```python
from build123d import *

# Parameters (mm, degrees)
SKETCH2_R          = 2.5
SKETCH2_R_2        = 2.2
SKETCH3_W          = 7.732538493
SKETCH3_H          = 7
CUT_EXTRUDE1_DEPTH = 5


with BuildPart() as part:
    # Sweep1: sweep along a path in Sketch1
    with BuildLine(Plane(origin=(0, 0, 0), x_dir=(0, 0, -1), z_dir=(1, 0, 0))) as sweep1_path:
        Line((0, 23), (-3, 23))
        ThreePointArc((-3, 23), (-15.57477634, 19.956594203), (-25.366269246, 11.5))
        ThreePointArc((-25.366269246, 11.5), (-31.811636627, 5.077357788), (-40, 1.10951216))
        ThreePointArc((-40, 1.10951216), (-43.826672111, 0.278791213), (-47.732538493, 0))
    # Sketch2 → Sweep1 (sweep)
    with BuildSketch(Plane.XY):
        with Locations((0, 23)):
            Circle(SKETCH2_R)
        with Locations((0, 23)):
            Circle(SKETCH2_R_2, mode=Mode.SUBTRACT)
    sweep(path=sweep1_path.line)

    # Sketch3 → Cut-Extrude1 (cut, symmetric)
    with BuildSketch(Plane(origin=(0, 0, 0), x_dir=(0, 0, -1), z_dir=(1, 0, 0))):
        with Locations((-43.866269246, 1)):
            Rectangle(SKETCH3_W, SKETCH3_H)
    extrude(amount=CUT_EXTRUDE1_DEPTH, both=True, mode=Mode.SUBTRACT)

    # Sketch4 → Revolve1 (revolve)
    with BuildSketch(Plane(origin=(0, 0, 0), x_dir=(0, 0, -1), z_dir=(1, 0, 0)), mode=Mode.PRIVATE) as revolve1_sk:
        with BuildLine():
            Line((0, 25.2), (0, 25.5))
            ThreePointArc((0, 25.5), (1.13447358, 25.928498418), (1.702386917, 27))
            Line((1.702386917, 27), (2, 26.962231588))
            ThreePointArc((2, 26.962231588), (1.332803452, 25.703408965), (0, 25.2))
        make_face()
    revolve(revolve1_sk.sketch.rotate(Axis((0, 23, 0), (0, 0, -1)), 90), axis=Axis((0, 23, 0), (0, 0, -1)))


solid = part.part
```
Source: CAD feature listing. Evaluate the final solid. Frame: model axes, mm. Round coordinates to 2 decimals unless told otherwise and drop trailing zeros. Write each loop counter-clockwise with the first axis right and the second up, starting at its lowest first coordinate (ties: lowest second). Pieces come first, ordered by that corner, then holes. Notation, with made-up numbers: M -14.5,71 L 24.5,71 A21 cw 24.5,108 Z; hole C -4,-11 d5. An arc over 180 degrees is marked long. Use CSV: the item, a comma, the result in double quotes. Start each with the question number.
Q1. Cut plane B-B on y = 19.5. Count the separate pieces of the cut face and the enclosed holes in it, plus the area to 3 significant figures.
Q2. Cut plane A-A on x = 0. Output: boundary loops of the cut face in (y, z), plus the area to 3 significant figures.
Q3. Pull-direction query (X, two-part tool) for faces 1 (the face through (-0.33, 25.48, 1.52)), 2 (the face through (-0.477, 20.852, 1.521)); classes: +X half, -X half, draft (parallel to the pull), parting line (faces both ways), or undercut.
Q4. Line query: line 1 (Y direction, x = 0, z = 2.1); line 2 (Z direction, x = -1, y = 15); line 3 (X direction, y = 17, z = 19). Output: solid intervals per line, ascending. Write a range as from..to.
Q5. First-contact query: P1, Ø1, axis at x = -2, z = 17.5, coming from the -Y side; P2, Ø4, axis at x = -2, y = 9, coming from the -Z side; P3, Ø4, axis at x = 0.5, z = 16, coming from the +Y side; P4, Ø3, axis at y = 12, z = 30.5, coming from the -X side. Flat tips, straight axial feed; report the tip coordinate or a pass-through.
Results found:
1,separate pieces,"2"
1,enclosed holes,"1"
1,area,"11.2 mm^2"
2,outline,"M -1.49,40 A30 ccw 10.05,23.33 A25 cw 20.5,3 L 20.5,0 A1.72 cw 19,-1.7 L 19.04,-2 A2.02 ccw 20.8,0 L 20.8,3 A25.3 ccw 10.22,23.58 A29.7 cw -1.18,40 Z; M 3.41,40 A25.3 ccw 12.78,27.16 A29.7 cw 25.2,3 L 25.2,0 A2.02 ccw 26.96,-2 L 27,-1.7 A1.72 cw 25.5,0 L 25.5,3 A30 ccw 12.95,27.4 A25 cw 3.73,40 Z"
2,area,"30.1 mm^2"
3,face 1,"parting line"
3,face 2,"undercut"
4,line 1,"20.5..20.8, 25.2..25.5"
4,line 2,"18.98..19.49, 25.08..25.52"
4,line 3,"-2.4..-2.09, 2.09..2.4"
5,P1,"y = 16.36"
5,P2,"z = 23.08"
5,P3,"y = 23.39"
5,P4,"through"
